from build123d import *

# Parameters (mm, degrees)
SKETCH_1_W          = 26
SKETCH_1_H          = 32
EXTRUDE_1_DEPTH     = 4
CHAMFER_1_SIZE      = 0.5
SKETCH_2_R          = 2.25
CUT_EXTRUDE_1_DEPTH = 42.424630354


with BuildPart() as part:
    # 草图1 → 凸台-拉伸1 (new body)
    with BuildSketch(Plane.XY):
        with Locations((13, 16)):
            Rectangle(SKETCH_1_W, SKETCH_1_H)
    extrude(amount=EXTRUDE_1_DEPTH)

    # 倒角1
    chamfer_1_edges = [part.edges().sort_by_distance(p)[0] for p in [
        (26, 16, 4),
        (13, 32, 4),
        (0, 16, 4),
        (13, 32, 0),
        (26, 16, 0),
        (13, 0, 0),
        (0, 16, 0),
        (13, 0, 4),
        (0, 32, 2),
        (26, 32, 2),
        (26, 0, 2),
        (0, 0, 2),
    ]]
    chamfer(chamfer_1_edges, length=CHAMFER_1_SIZE)

    # 草图2 → 切除-拉伸1 (cut, through all)
    with BuildSketch(Plane(origin=(0, 0, 0), x_dir=(-1, 0, 0), z_dir=(0, 0, -1))):
        with Locations((-19, 9)):
            Circle(SKETCH_2_R)
        with Locations((-19, 23)):
            Circle(SKETCH_2_R)
    extrude(amount=-CUT_EXTRUDE_1_DEPTH, mode=Mode.SUBTRACT)


solid = part.part
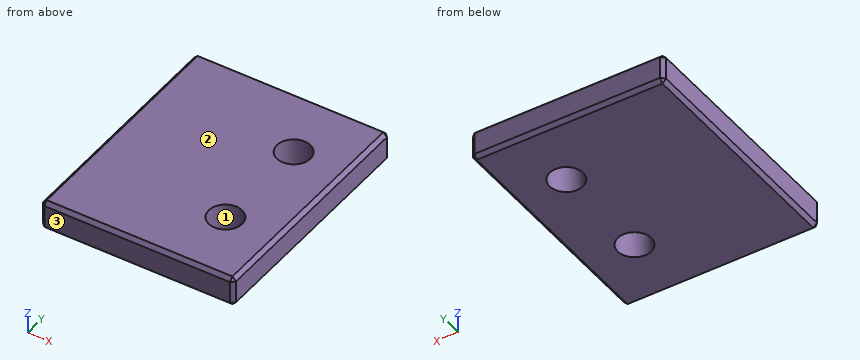
Input: part model. Units: mm. Frame: model coordinates. Face numbers are marked on the shaded views. Coordinates: 2 decimals unless noted, no trailing zeros. Order: outer loops, then holes, each group sorted by start corner. A loop starts at its lowest first (then second) coordinate and runs counter-clockwise, first axis right, second up. Notation, with made-up numbers: M -25.75,86 L -6.75,86 A31 cw -6.75,125 Z; hole C 28,-19 d8. An arc over 180 degrees is marked long. Write item = value, one per line. Start each with the question number.
(1) Line query: line 1 along Y through (x, z) = (19, 1.95); line 2 along Y through (x, z) = (17.5, 1.2); line 3 along X through (y, z) = (22, 1.85). Output: solid intervals per line, ascending. Write a range as [from, to].
(2) Pull-direction query (Y, two-part tool) for the marked faces 1, 2 and 3; classes: released by +Y, released by -Y, zero draft, split by the parting line, or undercut.
(3) Section B-B on z = 1.85. Output: boundary loops of the cut face in (x, y), and give its area (3 significant figures).
(4) Section C-C on y = 23. Output: boundary loops of the cut face in (x, z), and give its area (3 significant figures).
(5) First-contact query: P1, Ø12, axis at x = 18, y = 24.5, coming from the +Z side; P2, Ø4, axis at x = 19, y = 9, coming from the +Z side. Flat tips, straight axial feed; report the tip coordinate or a pass-through.
(6) Section A-A on x = 19. Output: boundary loops of the cut face in (y, z), and give its area (3 significant figures).
Result set:
q1.line_1 = [0, 6.75], [11.25, 20.75], [25.25, 32]
q1.line_2 = [0, 7.32], [10.68, 21.32], [24.68, 32]
q1.line_3 = [0, 16.98], [21.02, 26]
q2.face_1 = undercut
q2.face_2 = zero draft
q2.face_3 = released by -Y
q3.outline = M 0,0.5 L 0.5,0 L 25.5,0 L 26,0.5 L 26,31.5 L 25.5,32 L 0.5,32 L 0,31.5 Z; hole C 19,9 d4.5; hole C 19,23 d4.5
q3.area = 800 mm²
q4.outline = M 0,0.5 L 0.5,0 L 16.75,0 L 16.75,4 L 0.5,4 L 0,3.5 Z; M 21.25,0 L 25.5,0 L 26,0.5 L 26,3.5 L 25.5,4 L 21.25,4 Z
q4.area = 85.5 mm²
q5.P1 = 4
q5.P2 = through
q6.outline = M 0,0.5 L 0.5,0 L 6.75,0 L 6.75,4 L 0.5,4 L 0,3.5 Z; M 11.25,0 L 20.75,0 L 20.75,4 L 11.25,4 Z; M 25.25,0 L 31.5,0 L 32,0.5 L 32,3.5 L 31.5,4 L 25.25,4 Z
q6.area = 91.5 mm²
